For this review, take the finished solid that the model builds, in its own axes (mm). A direction names the side the tool comes from. Round coordinates to 2 decimals unless told otherwise and drop trailing zeros. Write each loop counter-clockwise with the first axis right and the second up, starting at its lowest first coordinate (ties: lowest second). Pieces come first, ordered by that corner, then holes. Notation, with made-up numbers: (70.5, -36.5) -> (97.5, -36.5) arc R19 cw to (97.5, -19.5) -> close; hole circle Ø7 at (-14.75, -33.75). An arc over 180 degrees is marked (long way). Write each question's results on one line, items separated by ' | '. Start each with the question number.
Item 1: The part is to be moulded in two halves that separate along Z. For faces 1 (the cylindrical face through (32.19, 14.47, -27.82)), 2 (the flat face through (0, 24, -24)), 3 (the cylindrical face through (94.806, 22.91, 35.934)), say which applies: +Z half, -Z half, draft (parallel to the pull), parting line (faces both ways), or undercut.
Item 2: Add section A-A (z = 0). State the section outline as (x, y) points, plus the area to 3 significant figures.
Item 3: Clearance check with flat-ended pins moving along their axes: pin 1 (5 mm diameter, centred on x = 33.5, z = 33.5, fed in from +Y); pin 2 (12 mm diameter, centred on x = 93, y = -39.5, fed in from -Z); pin 3 (6 mm diameter, centred on x = 102.5, z = -2.5, fed in from -Y); pin 4 (12 mm diameter, centred on y = -19, z = 31, fed in from -X). State where each tip first meets the part, or that it passes through.
Item 4: Tool access review of faces 4 (the flat face through (63.5, -13, -41)), 5 (the flat face through (127, -3.4, -31.4)): name each direction out of +Z, -Z, +X, -X, +Y, -Y from which nothing blocks a thin tool from reaching the whole face with its end or side.
Item 5: Add section C-C (x = 48.5). State the section outline as (y, z) points.
Item 6: Add section D-D (z = -36). State the section outline as (x, y) points, plus the area to 3 significant figures.
Item 7: To check wall thickness, follow line 1 along Z through (x, y) = (120, -1); line 2 along Z through (x, y) = (35, 0); line 3 along X through (y, z) = (34, -34). State the ranges of each line that lie inside material, in increasing order.
from build123d import *

# Parameters (mm, degrees)
F0_R     = 55.585182
F1_DEPTH = 63.5
F2_R     = 31.357467
F3_DEPTH = 63.5
F4_R     = 42.616489
F5_DEPTH = 63.5
F6_R     = 31.408113
F7_DEPTH = 63.5


with BuildPart() as f1:
    # F0 (on Right) → F1 (new body)
    with BuildSketch(Plane.YZ):
        Circle(F0_R)
    extrude(amount=F1_DEPTH)

    # F2 (on face) → F3 (cut)
    with BuildSketch(Plane.YZ.offset(63.5)):
        Circle(F2_R)
    extrude(amount=-F3_DEPTH, mode=Mode.SUBTRACT)

    # F4 (on face) → F5 (join)
    with BuildSketch(Plane.YZ.offset(63.5)):
        Circle(F4_R)
    extrude(amount=F5_DEPTH)

    # F6 (on face) → F7 (cut)
    with BuildSketch(Plane(origin=(63.5, 0, 0), x_dir=(0, -1, 0), z_dir=(-1, 0, 0))):
        Circle(F6_R)
    extrude(amount=-F7_DEPTH, mode=Mode.SUBTRACT)


solid = f1.part
Responses:
1) face 1: undercut | face 2: draft | face 3: parting line
2) outline: (0, -55.59) -> (63.5, -55.59) -> (63.5, -42.62) -> (127, -42.62) -> (127, -31.41) -> (63.5, -31.41) -> (63.5, -31.36) -> (0, -31.36) -> close; (0, 31.36) -> (63.5, 31.36) -> (63.5, 31.41) -> (127, 31.41) -> (127, 42.62) -> (63.5, 42.62) -> (63.5, 55.59) -> (0, 55.59) -> close | area: 4,500 mm^2
3) pin 1: stops at y = 46.14 | pin 2: stops at z = -26.34 | pin 3: stops at y = -42.62 | pin 4: stops at x = 0
4) face 4: +X | face 5: +Z, -Z, +X, +Y, -Y
5) outline: circle Ø111.17 at (0, 0); hole circle Ø62.71 at (0, 0)
6) outline: (0, -42.35) -> (63.5, -42.35) -> (63.5, -22.81) -> (127, -22.81) -> (127, 22.81) -> (63.5, 22.81) -> (63.5, 42.35) -> (0, 42.35) -> close | area: 8,280 mm^2
7) line 1: z = -42.6 to -31.39, 31.39 to 42.6 | line 2: z = -55.59 to -31.36, 31.36 to 55.59 | line 3: x = 0 to 63.5
